The listing builds one solid part. Answer for the finished solid, in the listing's coordinates (mm). A direction names the side the tool comes from. Coordinates: 2 decimals unless noted, no trailing zeros. Write each loop counter-clockwise with the first axis right and the second up, starting at its lowest first coordinate (ties: lowest second). Pieces come first, ordered by that corner, then holes.
from build123d import *

# Parameters (mm, degrees)
SKETCH1_R           = 1.5
BOSS_EXTRUDE1_DEPTH = 3


with BuildPart() as part:
    # Sketch1 → Boss-Extrude1 (new body)
    with BuildSketch(Plane.XY):
        Polygon((0, 17), (0, 22), (138, 22), (138, 17), (141, 17), (141, 7), (138, 7), (138, 0), (128, 0), (128, -3), (115, -3), (115, 0), (102, 0), (102, -3), (89, -3), (89, 0), (76, 0), (76, -3), (62, -3), (62, 0), (49, 0), (49, -3), (36, -3), (36, 0), (23, 0), (23, -3), (10, -3), (10, 0), (0, 0), (0, 7), (-3, 7), (-3, 17), align=None)
        with Locations((69, 15)):
            Circle(SKETCH1_R, mode=Mode.SUBTRACT)
    extrude(amount=BOSS_EXTRUDE1_DEPTH)


solid = part.part
Q1. Which of the six approach directions +Z, -Z, +X, -X, +Y, -Y give full straight-line access (tool end or side, diameter ignored) to faces 4 (the face through (30, 0, 1)), 5 (the face through (128, -1, 1)), 6 (the face through (139, 17, 1))?
Answers below:
face 4: +Z, -Z, -Y
face 5: +Z, -Z, +X, -Y
face 6: +Z, -Z, +X, +Y
Q2. Determine the mould class of faces 1 (the face through (49, -1, 1)), 2 (the face through (5, 0, 1)), 3 (the face through (0, 3, 1)) for opening direction X: released by +X, released by -X, zero draft, split by the parting line, or undercut.
Answers below:
face 1: undercut
face 2: zero draft
face 3: released by -X
Q3. Find the intervals of material crossed by probe 1 along Y at (x, z) = (69, 1.85); probe 2 along Y at (x, z) = (56.5, 2.05); probe 3 along X at (y, z) = (18, 1.8), in increasing order.
Answers below:
probe 1: y = -3 to 13.5, 16.5 to 22
probe 2: y = 0 to 22
probe 3: x = 0 to 138
Q4. The part is cut by section A-A, the plane y = 15. Write down the section's boundary in (x, z), then the cut area to 3 significant figures.
Answers below:
outline: (-3, 0) - (67.5, 0) - (67.5, 3) - (-3, 3) - close; (70.5, 0) - (141, 0) - (141, 3) - (70.5, 3) - close
area: 423 mm2
Q5. The part is cut by section D-D, the plane y = 4.5. Write down the section's boundary in (x, z).
Answers below:
outline: (0, 0) - (138, 0) - (138, 3) - (0, 3) - close
Q6. The part is cut by section C-C, the plane x = 69. Write down the section's boundary in (y, z).
Answers below:
outline: (-3, 0) - (13.5, 0) - (13.5, 3) - (-3, 3) - close; (16.5, 0) - (22, 0) - (22, 3) - (16.5, 3) - close
Q7. Given pin 1 (0.9 mm diameter, centred on x = 139, z = 1, fed in from -Y); pin 2 (0.9 mm diameter, centred on y = -2, z = 1.5, fed in from +X); pin 3 (1.5 mm diameter, centred on y = -1.5, z = 1, fed in from -X), each flat-ended and moving along its own axis, determine where each tip first touches the part or whether it passes through.
Answers below:
pin 1: stops at y = 7
pin 2: stops at x = 128
pin 3: stops at x = 10
